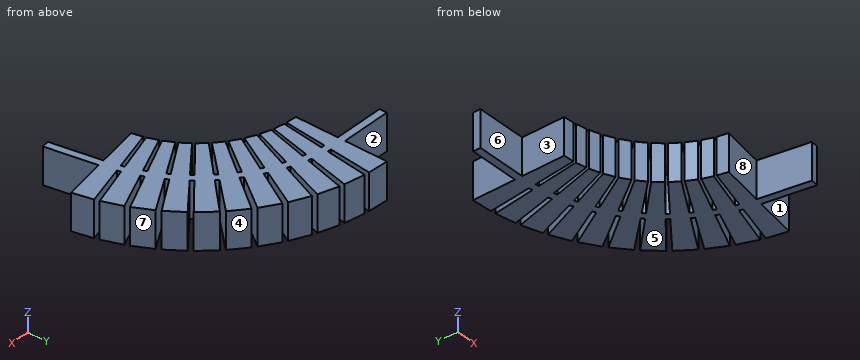
from build123d import *

# Parameters (mm, degrees)
AUFSATZ_LINEAR_AUSTRAGEN1_DEPTH = 5
AUFSATZ_LINEAR_AUSTRAGEN2_DEPTH = 5
KREISMUSTER1_COUNT              = 11
KREISMUSTER1_ANGLE              = 74
AUFSATZ_LINEAR_AUSTRAGEN4_DEPTH = 5
AUFSATZ_LINEAR_AUSTRAGEN3_DEPTH = 5
KREISMUSTER4_COUNT              = 11
KREISMUSTER4_ANGLE              = 74
SKIZZE5_W                       = 10
SKIZZE5_H                       = 2
AUFSATZ_LINEAR_AUSTRAGEN5_DEPTH = 13.6
SKIZZE6_W                       = 2
SKIZZE6_H                       = 10
AUFSATZ_LINEAR_AUSTRAGEN6_DEPTH = 13.6


with BuildPart() as part:
    # Skizze1 → Aufsatz-Linear austragen1 (new, symmetric)
    with BuildSketch(Plane.XY):
        with BuildLine():
            Line((0, 41), (0, 40))
            ThreePointArc((0, 40), (25.711504387, 30.641777725), (39.39231012, 6.945927107))
            Line((39.39231012, 6.945927107), (40.377117874, 7.119575284))
            ThreePointArc((40.377117874, 7.119575284), (26.354291997, 31.407822168), (0, 41))
        make_face()
    extrude(amount=AUFSATZ_LINEAR_AUSTRAGEN1_DEPTH, both=True)

    # Skizze2 → Aufsatz-Linear austragen2 (add, symmetric)
    with BuildSketch(Plane.XY):
        with BuildLine():
            Line((0, 41), (0, 52.6))
            Line((0, 52.6), (5.498197168, 52.311851696))
            Line((5.498197168, 52.311851696), (4.285666994, 40.77539771))
            ThreePointArc((4.285666994, 40.77539771), (2.145774206, 40.943810925), (0, 41))
        make_face()
    aufsatz_linear_austragen2 = extrude(amount=AUFSATZ_LINEAR_AUSTRAGEN2_DEPTH, both=True)

    # Kreismuster1: Aufsatz-Linear austragen2 ×11 about axis
    kreismuster1_axis = Axis((0, 0, 0), (0, 0, -1))
    for i in range(1, KREISMUSTER1_COUNT):
        add(aufsatz_linear_austragen2.rotate(kreismuster1_axis, i * KREISMUSTER1_ANGLE / (KREISMUSTER1_COUNT - 1)))

    # Skizze4 → Aufsatz-Linear austragen4 (add, symmetric)
    with BuildSketch(Plane.XY):
        with BuildLine():
            Line((0, 40), (0, 39))
            ThreePointArc((0, 39), (25.068716778, 29.875733282), (38.407502367, 6.772278929))
            Line((38.407502367, 6.772278929), (39.39231012, 6.945927107))
            ThreePointArc((39.39231012, 6.945927107), (25.711504387, 30.641777725), (0, 40))
        make_face()
    extrude(amount=AUFSATZ_LINEAR_AUSTRAGEN4_DEPTH, both=True)

    # Skizze3 → Aufsatz-Linear austragen3 (add, symmetric)
    with BuildSketch(Plane.XY):
        Polygon((4.181138531, 39.780875815), (0, 40), (0, 27.4), (2.864079894, 27.249899933), align=None)
    aufsatz_linear_austragen3 = extrude(amount=AUFSATZ_LINEAR_AUSTRAGEN3_DEPTH, both=True)

    # Kreismuster4: Aufsatz-Linear austragen3 ×11 about axis
    kreismuster4_axis = Axis((0, 0, 0), (0, 0, -1))
    for i in range(1, KREISMUSTER4_COUNT):
        add(aufsatz_linear_austragen3.rotate(kreismuster4_axis, i * KREISMUSTER4_ANGLE / (KREISMUSTER4_COUNT - 1)))

    # Skizze5 → Aufsatz-Linear austragen5 (add)
    with BuildSketch(Plane.ZY):
        with Locations((0, 40)):
            Rectangle(SKIZZE5_W, SKIZZE5_H)
    extrude(amount=AUFSATZ_LINEAR_AUSTRAGEN5_DEPTH)

    # Skizze6 → Aufsatz-Linear austragen6 (add)
    with BuildSketch(Plane(origin=(0, 0, 0), x_dir=(0.9848077530122074, 0.1736481776669343, 0), z_dir=(0.1736481776669343, -0.9848077530122074, 0))):
        with Locations((40, 0)):
            Rectangle(SKIZZE6_W, SKIZZE6_H)
    extrude(amount=AUFSATZ_LINEAR_AUSTRAGEN6_DEPTH)


solid = part.part
Verification items for the finished model (mm, model axes). Face numbers are marked on the shaded views. A direction names the side the tool comes from. Coordinates: 2 decimals unless noted, no trailing zeros. Loops run counter-clockwise (first coordinate to the right, second up) from the corner with the lowest first, then second, coordinate; pieces in that order, holes last. Notation, with made-up numbers: (46, 47) -> (102, 47) arc R24 ccw to (102, 69) -> close; hole circle Ø9 at (-29.5, -39.75). An arc over 180 degrees is marked (long way). Write each question's results on one line, items separated by ' | '.
Item 1: Tool access check on the marked faces 1, 2, 3, 4 and 5. Record the directions out of +Z, -Z, +X, -X, +Y, -Y that give a thin tool (end or side, any length) a straight path to the whole face; none if there is none.
Found:
face 1: +Z, -Z, +X | face 2: +Z, -Z, -X, +Y | face 3: +Z, -Z, -X, -Y | face 4: +Z, -Z, +X, +Y | face 5: -Z, +X, -X, +Y, -Y
Item 2: Material ranges on L1, parallel to X at y = 24.5, z = 0.25; L2, parallel to X at y = 41.5, z = 0.75; L3, parallel to X at y = 18, z = 1.75, recorded low to high.
Found:
L1: x = 12.2 to 13.14, 13.92 to 17.54, 18.46 to 22.85, 23.99 to 29.62, 30.34 to 38.91, 41.1 to 46.46 | L2: x = 0 to 4.36, 5.39 to 9.89, 10.96 to 15.76, 16.94 to 22.25, 23.58 to 29.71, 31.27 to 32.26 | L3: x = 20.62 to 21.76, 22.87 to 28.58, 30.2 to 38.96, 41.6 to 49.35
Item 3: Mould release check, pull along X, two halves, no side actions. Record for the marked faces 6, 7 and 8: +X half, -X half, draft (parallel to the pull), parting line (faces both ways), or undercut.
Found:
face 6: draft | face 7: +X half | face 8: undercut
Item 4: Section check A-A, the plane x = -4.5. Enter the section's corners in (y, z).
Found:
outline: (39, -5) -> (41, -5) -> (41, 5) -> (39, 5) -> close
Item 5: Gauge pin test, flat ends, axial feed: pin 1 (2 mm diameter, centred on x = 35, z = -0.5, fed in from -Y); pin 2 (1.5 mm diameter, centred on y = 12, z = 4, fed in from +X); pin 3 (3 mm diameter, centred on y = 45.5, z = -0.5, fed in from -X). Record the tip position at first contact, or that the pin passes through.
Found:
pin 1: stops at y = 6 | pin 2: stops at x = 51.31 | pin 3: stops at x = 0
